Geometry check sheet. Reference: the model listing, model coordinates, mm. A direction names the side the tool comes from. Give positions to 0.01 mm unless a question says otherwise; leave off trailing zeros. Loops run counter-clockwise (first coordinate to the right, second up) from the corner with the lowest first, then second, coordinate; pieces in that order, holes last. Notation, with made-up numbers: (-5, -22) - (6, -22) arc R17 ccw to (6, 0) - close; hole circle Ø5 at (71.25, -4.75). An arc over 180 degrees is marked (long way). One line per question, with ' | ' between items. Start each with the question number.
from build123d import *

# Parameters (mm, degrees)
SKETCH1_W               = 30
SKETCH1_H               = 25
SKETCH1_R               = 4
BOSS_EXTRUDE1_DEPTH     = 10
SKETCH2_W               = 30
SKETCH2_H               = 35
BOSS_EXTRUDE3_DEPTH     = 5
BOSS_EXTRUDE4_DEPTH     = 2.5
CUT_EXTRUDE1_DEPTH      = 26
CUT_EXTRUDE1_DEPTH_BACK = 6


with BuildPart() as part:
    # Sketch1 → Boss-Extrude1 (new body)
    with BuildSketch(Plane.XY):
        Rectangle(SKETCH1_W, SKETCH1_H)
        Circle(SKETCH1_R, mode=Mode.SUBTRACT)
    extrude(amount=BOSS_EXTRUDE1_DEPTH)

    # Sketch2 → Boss-Extrude3 (add)
    with BuildSketch(Plane.XZ.offset(12.5)):
        with Locations((0, 17.5)):
            Rectangle(SKETCH2_W, SKETCH2_H)
    extrude(amount=BOSS_EXTRUDE3_DEPTH)

    # Sketch7 → Boss-Extrude4 (add)
    with BuildSketch(Plane(origin=(15, 0, 0), x_dir=(0, 0, -1), z_dir=(1, 0, 0))):
        Polygon((-35, -12.5), (-10, 12.5), (-10, -12.5), align=None)
    boss_extrude4 = extrude(amount=-BOSS_EXTRUDE4_DEPTH)

    # Mirror1: Boss-Extrude4 across plane
    add(boss_extrude4.mirror(Plane(origin=(0, 0, 0), x_dir=(0, 0, 1), z_dir=(1, 0, 0))))

    # Sketch8 → Cut-Extrude1 (cut, two sides)
    with BuildSketch(Plane(origin=(0, -12.5, 0), x_dir=(1, 0, 0), z_dir=(0, 1, 0))) as cut_extrude1_sk:
        with BuildLine():
            Line((3.647363535, -16.948096307), (3.647363535, -27.842195287))
            ThreePointArc((3.647363535, -27.842195287), (0, -31.489558822), (-3.647363535, -27.842195287))
            Line((-3.647363535, -27.842195287), (-3.647363535, -16.948096307))
            ThreePointArc((-3.647363535, -16.948096307), (0, -13.300732772), (3.647363535, -16.948096307))
        make_face()
    extrude(amount=CUT_EXTRUDE1_DEPTH, mode=Mode.SUBTRACT)
    extrude(cut_extrude1_sk.sketch, amount=-CUT_EXTRUDE1_DEPTH_BACK, mode=Mode.SUBTRACT)


solid = part.part
(1) Section check C-C, the plane y = -15. Record the boundary of the cut face in (x, z), and give its area (3 significant figures).
(2) Section check A-A, the plane x = 0. Record the boundary of the cut face in (y, z), and give its area (3 significant figures).
(3) Mould release check, pull along X, two halves, no side actions. Record for faces 4 (the face through (0, 12.5, 5)), 5 (the face through (12.5, -5, 17)), 6 (the face through (15, -6, 13)): pulls with the +X half, pulls with the -X half, needs draft (parallel to the pull), parting line crosses it, or undercut.
(4) Material ranges on line 1 (X direction, y = -5.5, z = 14); line 2 (Y direction, x = 0, z = 4); line 3 (Z direction, x = 11.75, y = 7.5), recorded low to high.
(5) Section check B-B, the plane z = 26. Record the boundary of the cut face in (x, y), and give its area (3 significant figures).
(6) Tool access check on faces 1 (the face through (-13.8, -0.2, 22.7)), 2 (the face through (-3.647, -15, 22)), 3 (the face through (-12.5, -5, 17)). Record the directions out of +Z, -Z, +X, -X, +Y, -Y that give a thin tool (end or side, any length) a straight path to the whole face; none if there is none.
(7) Section check D-D, the plane y = 0. Record the boundary of the cut face in (x, z).
Numbers:
1) outline: (-15, 0) - (15, 0) - (15, 35) - (-15, 35) - close; hole (-3.65, 16.95) arc R3.65 ccw to (3.65, 16.95) - (3.65, 27.84) arc R3.65 ccw to (-3.65, 27.84) - close | area: 929 mm^2
2) outline: (-17.5, 0) - (-4, 0) - (-4, 10) - (-12.5, 10) - (-12.5, 13.3) - (-17.5, 13.3) - close; (-17.5, 31.49) - (-12.5, 31.49) - (-12.5, 35) - (-17.5, 35) - close; (4, 0) - (12.5, 0) - (12.5, 10) - (4, 10) - close | area: 254 mm^2
3) face 4: needs draft | face 5: undercut | face 6: pulls with the +X half
4) line 1: -15 to -12.5, 12.5 to 15 | line 2: -17.5 to -4, 4 to 12.5 | line 3: 0 to 10
5) outline: (-15, -17.5) - (-3.65, -17.5) - (-3.65, -12.5) - (-12.5, -12.5) - (-12.5, -3.5) - (-15, -3.5) - close; (3.65, -17.5) - (15, -17.5) - (15, -3.5) - (12.5, -3.5) - (12.5, -12.5) - (3.65, -12.5) - close | area: 159 mm^2
6) face 1: +Z, +X, -X, +Y | face 2: +Y, -Y | face 3: +Z, +Y
7) outline: (-15, 0) - (-4, 0) - (-4, 10) - (-12.5, 10) - (-12.5, 22.5) - (-15, 22.5) - close; (4, 0) - (15, 0) - (15, 22.5) - (12.5, 22.5) - (12.5, 10) - (4, 10) - close
